The model under review builds one solid part; all positions refer to its coordinate system, in mm. A direction names the side the tool comes from. Coordinates: 2 decimals unless noted, no trailing zeros. Loops run counter-clockwise (first coordinate to the right, second up) from the corner with the lowest first, then second, coordinate; pieces in that order, holes last. Notation, with made-up numbers: M -35.5,49 L 12.5,49 A25 ccw 12.5,77 Z; hole C 6.5,38.5 d7. An arc over 180 degrees is marked long. One line per item, written item: value.
```python
from build123d import *

# Parameters (mm, degrees)
F0_W      = 21.209
F0_H      = 21.209
F1_DEPTH  = 7.747
F2_R      = 5.08
F4_DEPTH  = 11.811
F6_DEPTH  = 8.1026
F7_R      = 15.113
F8_DEPTH  = 20.32
F9_R      = 10
F10_DEPTH = 9.017
F11_R     = 4.953
F12_DEPTH = 15.24
F13_R     = 6.477
F14_DEPTH = 1.0414


with BuildPart() as f1:
    # F0 (on Top) → F1 (new body)
    with BuildSketch(Plane.XY):
        Rectangle(F0_W, F0_H)
    extrude(amount=-F1_DEPTH)

    # F2
    f2_edges = [f1.edges().sort_by_distance(p)[0] for p in [
        (10.6045, -10.6045, -3.8735),
        (-10.6045, -10.6045, -3.8735),
        (-10.6045, 10.6045, -3.8735),
        (10.6045, 10.6045, -3.8735),
    ]]
    fillet(f2_edges, radius=F2_R)

    # F3 (on face) → F4 (join)
    with BuildSketch(Plane(origin=(0, 0, -7.747), x_dir=(1, 0, 0), z_dir=(0, 0, -1))):
        with BuildLine():
            Line((8.8138, -5.5245), (8.8138, 5.5245))
            ThreePointArc((8.8138, 5.5245), (7.850386, 7.850386), (5.5245, 8.8138))
            Line((5.5245, 8.8138), (-5.5245, 8.8138))
            ThreePointArc((-5.5245, 8.8138), (-7.850386, 7.850386), (-8.8138, 5.5245))
            Line((-8.8138, 5.5245), (-8.8138, -5.5245))
            ThreePointArc((-8.8138, -5.5245), (-7.850386, -7.850386), (-5.5245, -8.8138))
            Line((-5.5245, -8.8138), (5.5245, -8.8138))
            ThreePointArc((5.5245, -8.8138), (7.850386, -7.850386), (8.8138, -5.5245))
        make_face()
    extrude(amount=F4_DEPTH)

    # F5 (on face) → F6 (join)
    with BuildSketch(Plane(origin=(0, 0, -19.558), x_dir=(1, 0, 0), z_dir=(0, 0, -1))):
        Polygon((15.9385, -9.202097), (15.9385, 9.202097), (0, 18.404195), (-15.9385, 9.202097), (-15.9385, -9.202097), (0, -18.404195), align=None)
    extrude(amount=F6_DEPTH)

    # F7 (on face) → F8 (join)
    with BuildSketch(Plane(origin=(0, 0, -27.6606), x_dir=(1, 0, 0), z_dir=(0, 0, -1))):
        Circle(F7_R)
    extrude(amount=F8_DEPTH)

    # F9 (on face) → F10 (join)
    with BuildSketch(Plane(origin=(0, 0, -47.9806), x_dir=(1, 0, 0), z_dir=(0, 0, -1))):
        Circle(F9_R)
    extrude(amount=F10_DEPTH)

    # F11 (on face) → F12 (join)
    with BuildSketch(Plane(origin=(0, 0, -56.9976), x_dir=(1, 0, 0), z_dir=(0, 0, -1))):
        Circle(F11_R)
    extrude(amount=F12_DEPTH)

    # F13 (on face) → F14 (join)
    with BuildSketch(Plane(origin=(0, 0, -72.2376), x_dir=(1, 0, 0), z_dir=(0, 0, -1))):
        Circle(F13_R)
    extrude(amount=F14_DEPTH)

    # F15 (on Front) → F16 (revolve)
    with BuildSketch(Plane.XZ):
        Polygon((5.9055, -73.279), (0, -73.279), (0, -80.4418), (1.27, -80.4418), (4.6736, -78.613), align=None)
    revolve(axis=Axis((0, 0, -76.8604), (0, 0, -1)))


solid = f1.part
```
(1) Add section A-A on z = -24.5. State the section outline as (x, y) points.
Checks:
outline: M -15.94,-9.2 L 0,-18.4 L 15.94,-9.2 L 15.94,9.2 L 0,18.4 L -15.94,9.2 Z
(2) Add section C-C on x = 13. State the section outline as (y, z) points, then the cut area to 3 significant figures.
Checks:
outline: M -10.9,-27.66 L -7.71,-27.66 L -7.71,-47.98 L 7.71,-47.98 L 7.71,-27.66 L 10.9,-27.66 L 10.9,-19.56 L -10.9,-19.56 Z
area: 490 mm^2
(3) To check wall thickness, follow L1, parallel to Z at x = -4.5, y = 9; L2, parallel to Z at x = -2, y = -9; L3, parallel to Z at x = 2.5, y = -15. State the ranges of each line that lie inside material, in increasing order. Write a range as [from, to].
Checks:
L1: [-47.98, -19.56], [-7.75, 0]
L2: [-57, -19.56], [-7.75, 0]
L3: [-27.66, -19.56]
(4) Add section D-D on y = -8. State the section outline as (x, z) points.
Checks:
outline: M -15.94,-27.66 L -12.82,-27.66 L -12.82,-47.98 L -6,-47.98 L -6,-57 L 6,-57 L 6,-47.98 L 12.82,-47.98 L 12.82,-27.66 L 15.94,-27.66 L 15.94,-19.56 L 7.69,-19.56 L 7.69,-7.75 L 9.96,-7.75 L 9.96,0 L -9.96,0 L -9.96,-7.75 L -7.69,-7.75 L -7.69,-19.56 L -15.94,-19.56 Z
(5) Tool access review of faces 4 (the face through (7.9, -7.8, -13.6)), 5 (the face through (0, 8.814, -14)), 6 (the face through (9.156, 9.077, -3.928)), 7 (the face through (10.604, 0, -4)): name each direction out of +Z, -Z, +X, -X, +Y, -Y from which nothing blocks a thin tool from reaching the whole face with its end or side.
Checks:
face 4: +X, -Y
face 5: +X, -X, +Y
face 6: +Z, +X, +Y
face 7: +Z, +X, +Y, -Y
(6) Draft analysis for pull direction Z (two halves, no side actions). For faces 1 (the face through (-5, 2, -56.998)), 2 (the face through (6, -1, -73.279)), 3 (the face through (-15.938, 0, -24)), state which applies: pulls with the +Z half, pulls with the -Z half, needs draft (parallel to the pull), parting line crosses it, or undercut.
Checks:
face 1: undercut
face 2: pulls with the -Z half
face 3: needs draft
(7) Insertion check: pin 1 Ø8.5 at (x, z) = (-2.5, -2.5) entering from -Y; pin 2 Ø5.5 at (x, z) = (1.5, -15.5) entering from +Y; pin 3 Ø8.5 at (y, z) = (1, -5) entering from -X. Each pin has a flat end and moves straight along its axis. Give the tip position at first contact, or say it passes through.
Checks:
pin 1: y = -10.6
pin 2: y = 8.81
pin 3: x = -10.6
